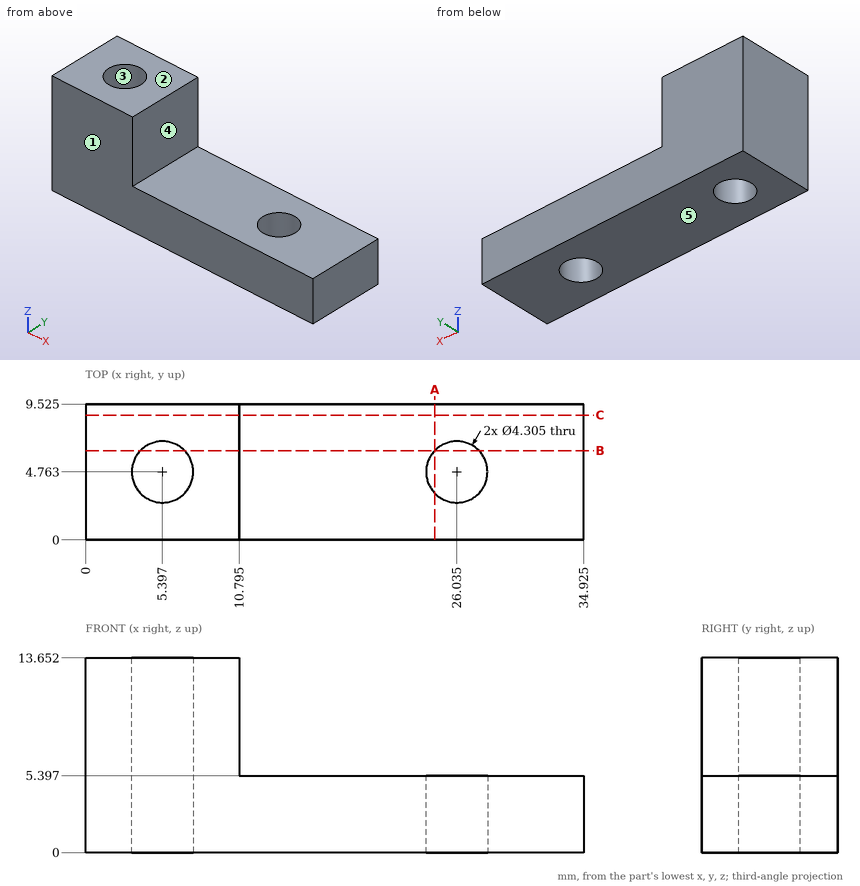
Source: three-view drawing plus pictorial views. Frame: mm from the lowest corner of the part. A direction names the side the tool comes from. Round coordinates to 2 decimals unless told otherwise and drop trailing zeros. Loops run counter-clockwise (first coordinate to the right, second up) from the corner with the lowest first, then second, coordinate; pieces in that order, holes last.
Q1. Section C-C on y = 8.75. Return loops of the section in (x, z) (1 decimal), plus the area to 3 significant figures.
Q2. Access query for the marked faces 4 and 5. Directions: +Z, -Z, +X, -X, +Y, -Y. A direction counts if a zero-diameter tool reaches every point of the face in a straight line with its end or side. Return the directions, or none.
Q3. Material intervals for L1, parallel to Z at x = 32.5, y = 8.25; L2, parallel to X at y = 4, z = 1 (1 decimal); L3, parallel to X at y = 1.25, z = 12.5 (1 decimal), sorted ascending.
Q4. Pull-direction query (Y, two-part tool) for the marked faces 1, 2 and 3; classes: released by +Y, released by -Y, zero draft, split by the parting line, or undercut.
Q5. Section B-B on y = 6.25. Return loops of the section in (x, z) (1 decimal).
Q6. Section A-A on x = 24.5. Return loops of the section in (y, z) (1 decimal).
Q7. Pin query (flat end, axial travel): P1, Ø3.5, axis at x = 26.04, y = 4.76, coming from the +Z side; P2, Ø4, axis at y = 5, z = 9, coming from the +X side (1 decimal). Return the tip coordinate at first contact, or that it passes through.
Evaluation:
1. outline: (0, 0) - (34.9, 0) - (34.9, 5.4) - (10.8, 5.4) - (10.8, 13.7) - (0, 13.7) - close
1. area: 278 mm2
2. face 4: +Z, +X, +Y, -Y
2. face 5: -Z, +X, -X, +Y, -Y
3. L1: z = 0 to 5.4
3. L2: x = 0 to 3.4, 7.4 to 24, 28 to 34.9
3. L3: x = 0 to 10.8
4. face 1: released by -Y
4. face 2: zero draft
4. face 3: undercut
5. outline: (0, 0) - (3.8, 0) - (3.8, 13.7) - (0, 13.7) - close; (7, 0) - (24.5, 0) - (24.5, 5.4) - (10.8, 5.4) - (10.8, 13.7) - (7, 13.7) - close; (27.6, 0) - (34.9, 0) - (34.9, 5.4) - (27.6, 5.4) - close
6. outline: (0, 0) - (3.3, 0) - (3.3, 5.4) - (0, 5.4) - close; (6.3, 0) - (9.5, 0) - (9.5, 5.4) - (6.3, 5.4) - close
7. P1: passes through
7. P2: stops at x = 10.8
